Build history of the part. All positions in model axes, mm. Give positions to 0.01 mm unless a question says otherwise; leave off trailing zeros. Order: outer loops, then holes, each group sorted by start corner. A loop starts at its lowest first (then second) coordinate and runs counter-clockwise, first axis right, second up. Notation, with made-up numbers: (61, 63.5) -> (119, 63.5) arc R34 cw to (119, 94.5) -> close; hole circle Ø11 at (-8, 51.25). An arc over 180 degrees is marked (long way). Use a Markdown table: item, result. Add a question column.
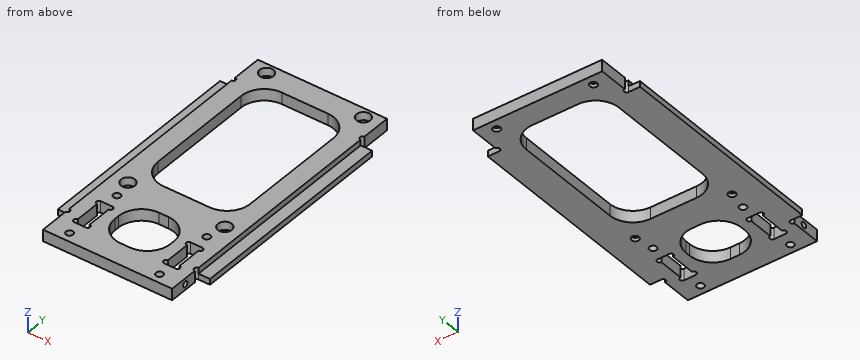
Autodesk Inventor part; units mm, degrees
ref_plane "YZ Plane" through (0, 0, 0) normal (1, 0, 0) x (0, 1, 0)
ref_plane "XZ Plane" through (0, 0, 0) normal (0, 1, 0) x (-1, 0, 0)
ref_plane "XY Plane" through (0, 0, 0) normal (0, 0, 1) x (1, 0, 0)
sketch "スケッチ1" plane through (0, 0, 0) normal (0, 0, 1) x (1, 0, 0)
  line L0 (-28, -61.25) -> (28, -61.25) construction
  line L1 (28, -61.25) -> (28, 61.25) construction
  line L2 (28, 61.25) -> (-28, 61.25) construction
  line L3 (-28, 61.25) -> (-28, -61.25) construction
  line L4 (-28, -61.25) -> (28, 61.25) construction
  line L5 (28, -61.25) -> (-28, 61.25) construction
  line L6 (-28, 48.35) -> (-28, 61.25)
  line L7 (-28, 61.25) -> (28, 61.25)
  line L8 (28, 61.25) -> (28, 48.35)
  line L9 (-28, 46.25) -> (-33, 46.25)
  line L10 (-33, 46.25) -> (-33, -46.25)
  line L11 (-33, -46.25) -> (-28, -46.25)
  line L12 (-28, -48.35) -> (-28, -61.25)
  line L13 (-28, -61.25) -> (28, -61.25)
  line L14 (28, -61.25) -> (28, -48.35)
  line L15 (28, 46.25) -> (33, 46.25)
  line L16 (33, 46.25) -> (33, -46.25)
  line L17 (33, -46.25) -> (28, -46.25)
  arc A0 (-28, 46.25) -> (-28, 48.35) centre (-28, 47.3) ccw
  arc A1 (-28, -48.35) -> (-28, -46.25) centre (-28, -47.3) ccw
  arc A2 (28, -46.25) -> (28, -48.35) centre (28, -47.3) ccw
  line L18 (0, 0) -> (0, 61.25) construction
  line L19 (0, 0) -> (28, 0) construction
  arc A3 (28, 48.35) -> (28, 46.25) centre (28, 47.3) ccw
  line L20 (-21, 56.95) -> (21, 56.95) construction
  line L21 (21, 56.95) -> (21, -22.05) construction
  line L22 (21, -22.05) -> (-21, -22.05) construction
  line L23 (-21, -22.05) -> (-21, 56.95) construction
  line L24 (-21, 56.95) -> (21, -22.05) construction
  line L25 (21, 56.95) -> (-21, -22.05) construction
  circle A4 centre (-21, 56.95) radius 1.6
  circle A5 centre (-21, -22.05) radius 1.6
  circle A6 centre (21, -22.05) radius 1.6
  circle A7 centre (21, 56.95) radius 1.6
  line L26 (-22, -36.25) -> (-17, -36.25) construction
  line L27 (-17, -36.25) -> (-17, -51.25) construction
  line L28 (-17, -51.25) -> (-22, -51.25) construction
  line L29 (-22, -51.25) -> (-22, -36.25) construction
  circle A8 centre (-19.5, -30.25) radius 1.55
  circle A9 centre (-19.5, -57.25) radius 1.55
  line L30 (-17, -43.75) -> (-22, -43.75) construction
  line L31 (-22, -26.25) -> (-17, -26.25) construction
  line L32 (-17, -26.25) -> (-17, -61.25) construction
  line L33 (-17, -61.25) -> (-22, -61.25) construction
  line L34 (-22, -61.25) -> (-22, -26.25) construction
  circle A10 centre (-19.5, -57.25) radius 3 construction
  line L35 (-16.95, -36.2) -> (-22.05, -36.2)
  line L36 (-22.05, -36.2) -> (-22.05, -51.3)
  line L37 (-22.05, -51.3) -> (-16.95, -51.3)
  line L38 (-16.95, -51.3) -> (-16.95, -36.2)
  circle A11 centre (-22.05, -37.25) radius 1.05
  circle A12 centre (-16.95, -37.25) radius 1.05
  circle A13 centre (-22.05, -50.25) radius 1.05
  circle A14 centre (-16.95, -50.25) radius 1.05
  circle A15 centre (19.5, -30.25) radius 1.55
  circle A16 centre (19.5, -57.25) radius 1.55
  line L39 (16.95, -36.2) -> (22.05, -36.2)
  line L40 (22.05, -36.2) -> (22.05, -51.3)
  line L41 (22.05, -51.3) -> (16.95, -51.3)
  line L42 (16.95, -51.3) -> (16.95, -36.2)
  circle A17 centre (22.05, -37.25) radius 1.05
  circle A18 centre (16.95, -37.25) radius 1.05
  circle A19 centre (22.05, -50.25) radius 1.05
  circle A20 centre (16.95, -50.25) radius 1.05
  point P0 (0, 17.45)
  point P1 (0, 17.45)
  point P2 (0, 0)
  point P3 (-19.5, -43.75)
  point P4 (-19.5, -26.25)
  dimension "d93" = 2.1
  dimension "d9" = 56
  dimension "d12" = 122.5
  dimension "d13" = 15
  dimension "d39" = 15
  dimension "d40" = 1.05
  dimension "d41" = 5
  dimension "d52" = 3.2
  dimension "d53" = 42
  dimension "d54" = 79
  dimension "d55" = 4.3
  dimension "d73" = 35
  dimension "d83" = 5
  dimension "d87" = 3.1
  dimension "d88" = 10
  dimension "d89" = 27
  dimension "d90" = 6
  dimension "d91" = 22
  dimension "d92" = 0.05
extrude "押し出し1" add sketch "スケッチ1" along normal blind 5
sketch "スケッチ2" plane through (0, 0, 5) normal (0, 0, 1) x (1, 0, 0)
  line L0 (-28, 61.25) -> (-28, 48.35)
  line L1 (28, 61.25) -> (-28, 61.25)
  line L2 (-67.7785, 47.5) -> (-28, 47.5)
  line L3 (-28, 47.5) -> (-28, -47.5)
  line L4 (-28, -47.5) -> (-67.7785, -47.5)
  line L5 (-67.7785, -47.5) -> (-67.7785, 47.5)
  line L6 (67.7785, 47.5) -> (28, 47.5)
  line L7 (28, 47.5) -> (28, -47.5)
  line L8 (28, -47.5) -> (67.7785, -47.5)
  line L9 (67.7785, -47.5) -> (67.7785, 47.5)
  line L10 (0, 0) -> (0, 61.25) construction
  line L11 (0, 0) -> (33, 0) construction
  line L12 (33, 46.25) -> (33, -46.25) construction
  dimension "d106" = 95
extrude "押し出し2" cut sketch "スケッチ2" against normal blind 2.5
sketch "スケッチ4" plane through (0, 0, 5) normal (0, 0, 1) x (1, 0, 0)
  line L0 (28, 61.25) -> (-28, 61.25)
  line L1 (-28, 61.25) -> (-28, 48.35)
  line L2 (-28, -61.25) -> (28, -61.25)
  line L3 (-16.95, -51.3) -> (-22.05, -51.3)
  arc A0 (-22.05, -49.2) -> (-22.05, -51.3) centre (-22.05, -50.25) ccw
  line L4 (-22.05, -49.2) -> (-22.05, -38.3)
  arc A1 (-22.05, -36.2) -> (-22.05, -38.3) centre (-22.05, -37.25) ccw
  line L5 (-22.05, -36.2) -> (-16.95, -36.2)
  arc A2 (-16.95, -38.3) -> (-16.95, -36.2) centre (-16.95, -37.25) ccw
  line L6 (-16.95, -38.3) -> (-16.95, -49.2)
  arc A3 (-16.95, -51.3) -> (-16.95, -49.2) centre (-16.95, -50.25) ccw
  circle A4 centre (-19.5, -30.25) radius 1.55
  line L7 (-20, 51.25) -> (20, 51.25)
  line L8 (20, 51.25) -> (20, -16.25)
  line L9 (20, -16.25) -> (-20, -16.25)
  line L10 (-20, -16.25) -> (-20, 51.25)
  line L11 (-12, -29.25) -> (12, -29.25)
  line L12 (12, -29.25) -> (12, -51.25)
  line L13 (12, -51.25) -> (-12, -51.25)
  line L14 (-12, -51.25) -> (-12, -29.25)
  line L15 (-16.95, -36.25) -> (-22.05, -36.25) construction
  arc A5 (-22.05, -36.25) -> (-22, -38.2487) centre (-22.05, -37.25) ccw construction
  line L16 (-22, -38.2487) -> (-22, -49.2513) construction
  arc A6 (-22, -49.2513) -> (-22.05, -51.25) centre (-22.05, -50.25) ccw construction
  line L17 (-22.05, -51.25) -> (-16.95, -51.25) construction
  arc A7 (-16.95, -51.25) -> (-17, -49.2513) centre (-16.95, -50.25) ccw construction
  line L18 (-17, -49.2513) -> (-17, -38.2487) construction
  arc A8 (-17, -38.2487) -> (-16.95, -36.25) centre (-16.95, -37.25) ccw construction
  point P0 (0, 0)
  point P1 (0, 51.25)
  point P2 (0, -16.25)
  point P3 (0, -29.25)
  dimension "d94" = 8
  dimension "d95" = 10
  dimension "d96" = 14
  dimension "d97" = 0.05
  dimension "d98" = 5
  dimension "d99" = 10
  dimension "d100" = 13
extrude "押し出し4" cut sketch "スケッチ4" against normal blind 10 contours L7 L8 L9 L10 | L11 L12 L13 L14
fillet "フィレット2" radius 10 8 edges at (-12, -51.25, 2.5) (-12, -29.25, 2.5) (12, -29.25, 2.5) (12, -51.25, 2.5) (-20, -16.25, 2.5) (-20, 51.25, 2.5) (20, 51.25, 2.5) (20, -16.25, 2.5)
sketch "スケッチ6" plane through (0, 0, 5) normal (0, 0, 1) x (1, 0, 0)
  circle A0 centre (-21, 57) radius 3
  circle A1 centre (-21, -22) radius 3
  line L0 (0, 0) -> (0, 20)
  circle A2 centre (21, 57) radius 3
  circle A3 centre (21, -22) radius 3
  dimension "d107" = 6
  dimension "d108" = 6
  dimension "d109" = 79
  dimension "d110" = 57
  dimension "d111" = 21
  dimension "d112" = 20
extrude "押し出し5" cut sketch "スケッチ6" against normal blind 3.5
sketch "スケッチ7" plane through (28, -61.25, 0) normal (1, 0, 0) x (0, 0, -1)
  line L0 (0, 0) -> (-5, 0)
  line L1 (-5, 0) -> (-5, 12.9)
  point P0 (0, 61.25)
  point P1 (-2.5, 7.5)
  dimension "d115" = 7.5
  dimension "d116" = 5
  dimension "d117" = 2.5
sketch "スケッチ8" plane through (-28, -61.25, 0) normal (-1, 0, 0) x (0, 0, 1)
  line L0 (0, 0) -> (5, 0)
  line L1 (5, 12.9) -> (5, 0)
  point P0 (0, 61.25)
  point P1 (2.5, 7.5)
  dimension "d118" = 7.5
  dimension "d119" = 2.5
hole "穴1" at (-28, -53.75, 2.5) direction (1, 0, 0) diameter 2.459 depth 12
hole "穴2" at (28, -53.75, 2.5) direction (-1, 0, 0) diameter 2.459 depth 12
equation "\"d12\" = d19"
equation "\"d13\" = d26"
equation "\"d39\" = d27"
equation "\"d73\" = d1_1_2_3 + 2 * d2_1"
equation "\"d88\" = d2_1"
equation "\"d99\" = d95"
properties part number "コックピット_2_サブフレーム_2" material "アセタール樹脂、黒"
(1) Band-saw the part on A-A on y = 17.5. Give the cut face in (x, z), plus the area to 3 significant figures.
(2) Wall check: probe 1 along X at (y, z) = (-39, 2.2); probe 2 along Y at (x, z) = (-1.5, 2.95); probe 3 along X at (y, z) = (-22.05, 0.9). Give the ranges that are in metal, low to high.
(3) Band-saw the part on C-C on y = -34. Give the cut face in (x, z), plus the area to 3 significant figures.
(4) Pin check, flat tips, straight feed: pin 1 Ø0.7 at (y, z) = (-54, 2) entering from +X; pin 2 Ø3 at (x, z) = (31.5, 1.5) entering from -Y; pin 3 Ø4 at (x, y) = (31, -3.5) entering from +Z. Stop position of each tip, or through.
(5) Band-saw the part on B-B on x = 14. Give the cut face in (y, z).
Response:
| question | item | result |
|---|---|---|
| 1 | outline | (-33, 0) -> (-20, 0) -> (-20, 5) -> (-28, 5) -> (-28, 2.5) -> (-33, 2.5) -> close; (20, 0) -> (33, 0) -> (33, 2.5) -> (28, 2.5) -> (28, 5) -> (20, 5) -> close |
| 1 | area | 105 mm² |
| 2 | probe 1 | x = -33 to -22.05, -16.95 to -12, 12 to 16.95, 22.05 to 33 |
| 2 | probe 2 | y = -61.25 to -51.25, -29.25 to -16.25, 51.25 to 61.25 |
| 2 | probe 3 | x = -33 to -22.6, -19.4 to 19.4, 22.6 to 33 |
| 3 | outline | (-33, 0) -> (-10.51, 0) -> (-10.51, 5) -> (-28, 5) -> (-28, 2.5) -> (-33, 2.5) -> close; (10.51, 0) -> (33, 0) -> (33, 2.5) -> (28, 2.5) -> (28, 5) -> (10.51, 5) -> close |
| 3 | area | 200 mm² |
| 4 | pin 1 | stops at x = 16 |
| 4 | pin 2 | stops at y = -46.25 |
| 4 | pin 3 | stops at z = 2.5 |
| 5 | outline | (-61.25, 0) -> (-15.42, 0) -> (-15.42, 5) -> (-61.25, 5) -> close; (50.42, 0) -> (61.25, 0) -> (61.25, 5) -> (50.42, 5) -> close |
